Design review of the part built by this model. Coordinates are the model's own, in mm. Face numbers are marked on the shaded views. A direction names the side the tool comes from. Give positions to 0.01 mm unless a question says otherwise; leave off trailing zeros. Order: outer loops, then holes, each group sorted by start corner. A loop starts at its lowest first (then second) coordinate and runs counter-clockwise, first axis right, second up. Notation, with made-up numbers: M -32,26 L 11,26 A30 ccw 11,54 Z; hole C 46.25,64.5 d7. An arc over 180 degrees is marked long. Answer as a JSON object with one key per item and string values.
from build123d import *

# Parameters (mm, degrees)
SKETCH1_W                 = 37.5
SKETCH1_H                 = 36.5
BOSS_EXTRUDE1_DEPTH       = 5
SHELL1_T                  = 5
BOSS_EXTRUDE2_START       = -2
BOSS_EXTRUDE2_OUTLINE_W   = 8
BOSS_EXTRUDE2_OUTLINE_H   = 8
BOSS_EXTRUDE2_OUTLINE_R   = 1.75
BOSS_EXTRUDE2_OUTLINE_W_2 = 37.5
BOSS_EXTRUDE2_OUTLINE_H_2 = 36.5
BOSS_EXTRUDE2_OUTLINE_W_3 = 35.5
BOSS_EXTRUDE2_OUTLINE_H_3 = 34.752631578
BOSS_EXTRUDE2_DEPTH       = 2
SKETCH3_W                 = 5
SKETCH3_H                 = 4
SKETCH3_H_2               = 14
CUT_EXTRUDE2_DEPTH        = 3
FILLET1_R                 = 2


# Read off the part's stored shape, not the designer's step: Boss-Extrude2
with BuildPart() as part:
    # Sketch1 → Boss-Extrude1 (new body)
    with BuildSketch(Plane.XY):
        with Locations((18.75, -18.25)):
            Rectangle(SKETCH1_W, SKETCH1_H)
    extrude(amount=BOSS_EXTRUDE1_DEPTH)

    # Shell1
    shell1_openings = [part.faces().sort_by_distance(p)[0] for p in [
        (18.75, -18.25, 0),
        (18.75, -18.25, 5),
    ]]
    offset(amount=SHELL1_T, openings=shell1_openings, kind=Kind.INTERSECTION)

    # Boss-Extrude2 outline → Boss-Extrude2 (add)
    # profile 1 of 3: a face of its own
    with BuildSketch(Plane(origin=(0, 0, 0), x_dir=(-1, 0, 0), z_dir=(0, 0, -1)).offset(BOSS_EXTRUDE2_START)):
        with Locations((-18.75, 9)):
            Rectangle(BOSS_EXTRUDE2_OUTLINE_W, BOSS_EXTRUDE2_OUTLINE_H)
        with Locations((-18.75, 9)):
            Circle(BOSS_EXTRUDE2_OUTLINE_R, mode=Mode.SUBTRACT)
    # profile 2 of 3: a face of its own
    with BuildSketch(Plane(origin=(0, 0, 0), x_dir=(-1, 0, 0), z_dir=(0, 0, -1)).offset(BOSS_EXTRUDE2_START)):
        with Locations((-18.75, -45.5)):
            Rectangle(BOSS_EXTRUDE2_OUTLINE_W, BOSS_EXTRUDE2_OUTLINE_H)
        with Locations((-18.75, -45.5)):
            Circle(BOSS_EXTRUDE2_OUTLINE_R, mode=Mode.SUBTRACT)
    # profile 3 of 3: a face of its own
    with BuildSketch(Plane(origin=(0, 0, 0), x_dir=(-1, 0, 0), z_dir=(0, 0, -1)).offset(BOSS_EXTRUDE2_START)):
        with Locations((-18.75, -18.25)):
            Rectangle(BOSS_EXTRUDE2_OUTLINE_W_2, BOSS_EXTRUDE2_OUTLINE_H_2)
        with Locations((-18.75, -18.25)):
            Rectangle(BOSS_EXTRUDE2_OUTLINE_W_3, BOSS_EXTRUDE2_OUTLINE_H_3, mode=Mode.SUBTRACT)
    extrude(amount=BOSS_EXTRUDE2_DEPTH)

    # Sketch3 → Cut-Extrude2 (cut)
    with BuildSketch(Plane.XY.offset(5)):
        with Locations((-2.5, -9)):
            Rectangle(SKETCH3_W, SKETCH3_H)
        with Locations((-2.5, -27.5)):
            Rectangle(SKETCH3_W, SKETCH3_H)
        with Locations((40, -18.25)):
            Rectangle(SKETCH3_W, SKETCH3_H_2)
    extrude(amount=-CUT_EXTRUDE2_DEPTH, mode=Mode.SUBTRACT)

    # Fillet1
    fillet1_edges = [part.edges().sort_by_distance(p)[0] for p in [
        (0, 0, 3.5),
        (0, -36.5, 3.5),
        (22.75, -41.5, 1),
        (22.75, 5, 1),
        (22.75, 13, 1),
        (14.75, 13, 1),
        (14.75, 5, 1),
        (14.75, -41.5, 1),
        (14.75, -49.5, 1),
        (22.75, -49.5, 1),
    ]]
    fillet(fillet1_edges, radius=FILLET1_R)


solid = part.part
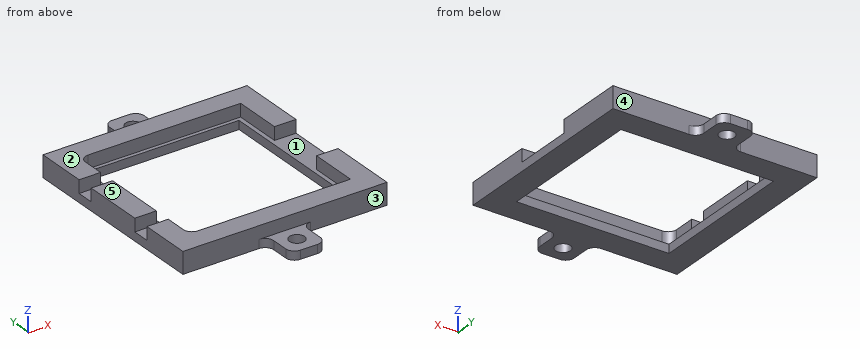
(1) To check wall thickness, follow L1, parallel to Y at x = -0.5, z = 4.65; L2, parallel to Y at x = 18.75, z = 0.55; L3, parallel to X at y = -34, z = 4.4. State the ranges of each line that lie inside material, in increasing order. Write a range as from..to.
Checked values:
{"L1": "y = -41.5..-29.5, -25.5..-11, -7..5", "L2": "y = -49.5..-47.25, -43.75..-35.63, -0.87..7.25, 10.75..13", "L3": "x = -5..0, 37.5..42.5"}
(2) We need section B-B (y = -18). Write out the cut boundary in (x, z).
Checked values:
{"outline": "M -5,0 L 1,0 L 1,2 L 0,2 L 0,5 L -5,5 Z; M 36.5,0 L 42.5,0 L 42.5,2 L 36.5,2 Z"}
(3) We need section A-A (x = 18.75). Write out the cut boundary in (y, z), plus the area to 3 significant figures.
Checked values:
{"outline": "M -49.5,0 L -47.25,0 L -47.25,2 L -49.5,2 Z; M -43.75,0 L -35.63,0 L -35.63,2 L -36.5,2 L -36.5,5 L -41.5,5 L -41.5,2 L -43.75,2 Z; M -0.87,0 L 7.25,0 L 7.25,2 L 5,2 L 5,5 L 0,5 L 0,2 L -0.87,2 Z; M 10.75,0 L 13,0 L 13,2 L 10.75,2 Z", "area": "71.5 mm^2"}
(4) Tool access review of the marked faces 4 and 5: name each direction out of +Z, -Z, +X, -X, +Y, -Y from which nothing blocks a thin tool from reaching the whole face with its end or side.
Checked values:
{"face 4": "+Z, +Y", "face 5": "+Z, +X, -X, +Y, -Y"}
(5) Insertion check: pin 1 (1.6 mm diameter, centred on y = 9.5, z = 1.5, fed in from +X); pin 2 (1.5 mm diameter, centred on x = -1.5, z = 3.5, fed in from +Y); pin 3 (2 mm diameter, centred on y = 10, z = 1, fed in from -X). Each pin has a flat end and moves straight along its axis. Give the tip position at first contact, or say it passes through.
Checked values:
{"pin 1": "stops at x = 22.75", "pin 2": "stops at y = 5", "pin 3": "stops at x = 14.75"}
(6) Draft analysis for pull direction Y (two halves, no side actions). For the marked faces 1, 2 and 3, state which applies: +Y half, -Y half, draft (parallel to the pull), parting line (faces both ways), or undercut.
Checked values:
{"face 1": "undercut", "face 2": "draft", "face 3": "-Y half"}
(7) We need section D-D (x = 31). Write out the cut boundary in (y, z).
Checked values:
{"outline": "M -41.5,0 L -35.63,0 L -35.63,2 L -36.5,2 L -36.5,5 L -41.5,5 Z; M -0.87,0 L 5,0 L 5,5 L 0,5 L 0,2 L -0.87,2 Z"}
(8) We need section C-C (z = 0.8). Write out the cut boundary in (x, y).
Checked values:
{"outline": "M -5,-41.5 L 12.75,-41.5 A2 cw 14.75,-43.5 L 14.75,-47.5 A2 ccw 16.75,-49.5 L 20.75,-49.5 A2 ccw 22.75,-47.5 L 22.75,-43.5 A2 cw 24.75,-41.5 L 42.5,-41.5 L 42.5,5 L 24.75,5 A2 cw 22.75,7 L 22.75,11 A2 ccw 20.75,13 L 16.75,13 A2 ccw 14.75,11 L 14.75,7 A2 cw 12.75,5 L -5,5 Z; hole M 1,-35.63 L 36.5,-35.63 L 36.5,-0.87 L 1,-0.87 Z; hole C 18.75,-45.5 d3.5; hole C 18.75,9 d3.5"}
